The listing builds one solid part. Answer for the finished solid, in the listing's coordinates (mm). Face numbers are marked on the shaded views. A direction names the side the tool comes from. Round coordinates to 2 decimals unless told otherwise and drop trailing zeros. Loops run counter-clockwise (first coordinate to the right, second up) from the corner with the lowest first, then second, coordinate; pieces in that order, holes last. Notation, with made-up numbers: (32.25, 62) -> (44.25, 62) arc R29 ccw to (44.25, 93) -> close; hole circle Ø1 at (45.5, 44). An arc over 180 degrees is marked (long way). One line per question, with ' | ' between items.
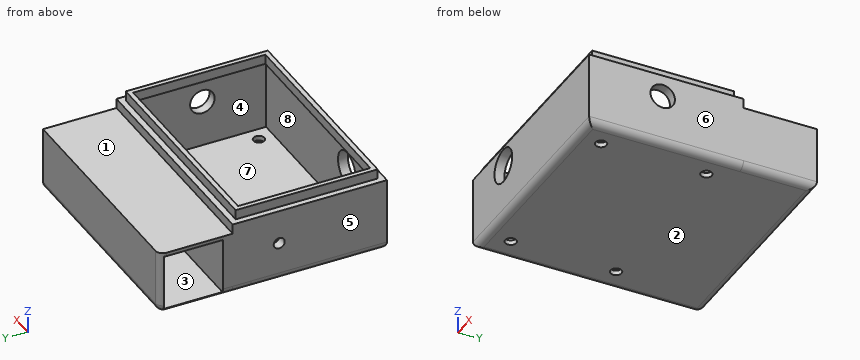
from build123d import *

# Parameters (mm, degrees)
SKETCH3_W           = 92
SKETCH3_H           = 63
SKETCH3_R           = 2.25
BOSS_EXTRUDE3_DEPTH = 30
SKETCH4_W           = 84
SKETCH4_H           = 55
CUT_EXTRUDE1_DEPTH  = 28
FILLET1_R           = 3
SKETCH5_W           = 87
SKETCH5_H           = 58
BOSS_EXTRUDE4_DEPTH = 4
SKETCH7_W           = 83
SKETCH7_H           = 54
CUT_EXTRUDE4_DEPTH  = 27
SKETCH9_R           = 7
CUT_EXTRUDE6_DEPTH  = 27
SKETCH11_R          = 5
CUT_EXTRUDE7_DEPTH  = 27
SKETCH12_R          = 2.25
CUT_EXTRUDE8_DEPTH  = 10
SKETCH13_W          = 92
SKETCH13_H          = 26
BOSS_EXTRUDE6_DEPTH = 30
SKETCH14_W          = 23
SKETCH14_H          = 24
CUT_EXTRUDE9_DEPTH  = 90
FILLET3_R           = 3
FILLET4_R           = 3


with BuildPart() as part:
    # Sketch3 → Boss-Extrude3 (new body)
    with BuildSketch(Plane.XY):
        with Locations((46, 31.5)):
            Rectangle(SKETCH3_W, SKETCH3_H)
        with Locations((82, 53)):
            Circle(SKETCH3_R, mode=Mode.SUBTRACT)
        with Locations((82, 10)):
            Circle(SKETCH3_R, mode=Mode.SUBTRACT)
        with Locations((10.5, 10)):
            Circle(SKETCH3_R, mode=Mode.SUBTRACT)
        with Locations((10.5, 53)):
            Circle(SKETCH3_R, mode=Mode.SUBTRACT)
    extrude(amount=BOSS_EXTRUDE3_DEPTH)

    # Sketch4 → Cut-Extrude1 (cut)
    with BuildSketch(Plane.XY.offset(30)):
        with Locations((46, 31.5)):
            Rectangle(SKETCH4_W, SKETCH4_H)
    extrude(amount=-CUT_EXTRUDE1_DEPTH, mode=Mode.SUBTRACT)

    # Fillet1
    fillet1_edges = [part.edges().sort_by_distance(p)[0] for p in [
        (92, 31.5, 0),
        (46, 0, 0),
        (0, 31.5, 0),
    ]]
    fillet(fillet1_edges, radius=FILLET1_R)

    # Sketch5 → Boss-Extrude4 (add)
    with BuildSketch(Plane.XY.offset(30)):
        with Locations((46, 31.5)):
            Rectangle(SKETCH5_W, SKETCH5_H)
    extrude(amount=BOSS_EXTRUDE4_DEPTH)

    # Sketch7 → Cut-Extrude4 (cut)
    with BuildSketch(Plane.XY.offset(34)):
        with Locations((46, 31.5)):
            Rectangle(SKETCH7_W, SKETCH7_H)
    extrude(amount=-CUT_EXTRUDE4_DEPTH, mode=Mode.SUBTRACT)

    # Sketch9 → Cut-Extrude6 (cut)
    with BuildSketch(Plane.XZ):
        with Locations(Location((24, 22, 0), (0, 0, 270))):
            Circle(SKETCH9_R)
    extrude(amount=-CUT_EXTRUDE6_DEPTH, mode=Mode.SUBTRACT)

    # Sketch11 → Cut-Extrude7 (cut)
    with BuildSketch(Plane(origin=(92, 0, 0), x_dir=(0, 0, -1), z_dir=(1, 0, 0))):
        with Locations((-21, 30)):
            Circle(SKETCH11_R)
    extrude(amount=-CUT_EXTRUDE7_DEPTH, mode=Mode.SUBTRACT)

    # Sketch12 → Cut-Extrude8 (cut)
    with BuildSketch(Plane.ZY):
        with Locations((16, 44)):
            Circle(SKETCH12_R)
    extrude(amount=-CUT_EXTRUDE8_DEPTH, mode=Mode.SUBTRACT)

    # Sketch13 → Boss-Extrude6 (add)
    with BuildSketch(Plane(origin=(0, 63, 0), x_dir=(1, 0, 0), z_dir=(0, 1, 0))):
        with Locations((46, -13)):
            Rectangle(SKETCH13_W, SKETCH13_H)
    extrude(amount=BOSS_EXTRUDE6_DEPTH)

    # Sketch14 → Cut-Extrude9 (cut)
    with BuildSketch(Plane.ZY):
        with Locations((13, 79)):
            Rectangle(SKETCH14_W, SKETCH14_H)
    extrude(amount=-CUT_EXTRUDE9_DEPTH, mode=Mode.SUBTRACT)

    # Fillet3
    fillet3_edges = [part.edges().sort_by_distance(p)[0] for p in [
        (46, 93, 0),
        (92, 78, 0),
    ]]
    fillet(fillet3_edges, radius=FILLET3_R)

    # Fillet4
    # the kernel refuses this fillet: 3 mm, written as the material it takes off along each edge
    with BuildSketch(Plane(origin=(0, 93, 33.5), x_dir=(0, -1, 0), z_dir=(0, 0, -1))) as fillet4_piece_1:
        with BuildLine():
            CenterArc((FILLET4_R, -FILLET4_R), FILLET4_R, 90, 90)
            Line((0, -FILLET4_R), (0, 0))
            Line((0, 0), (FILLET4_R, 0))
        make_face()
    extrude(amount=30.5, mode=Mode.SUBTRACT)
    with BuildSketch(Plane(origin=(0, 55.5, 0), x_dir=(0, 0, 1), z_dir=(0, 1, 0))) as fillet4_piece_2:
        with BuildLine():
            CenterArc((FILLET4_R, FILLET4_R), FILLET4_R, 180, 90)
            Line((0, FILLET4_R), (0, 0))
            Line((0, 0), (FILLET4_R, 0))
        make_face()
    extrude(amount=34.5, mode=Mode.SUBTRACT)
    with BuildSketch(Plane(origin=(0, 90, 3), x_dir=(0, 1, 0), z_dir=(0, 0, 1))) as fillet4_piece_3:
        with BuildLine():
            CenterArc((3 - FILLET4_R, -FILLET4_R), FILLET4_R, 0, 90)
            Line((3, -FILLET4_R), (3, 0))
            Line((3, 0), (3 - FILLET4_R, 0))
        make_face()
    revolve(axis=Axis((0, 90, 3), (-1, 0, 0)), revolution_arc=90, mode=Mode.SUBTRACT)


solid = part.part
Q1. A cutting plane is placed at D-D on z = 5. Give the vertices of the cut face in (x, y).
Numbers:
outline: (0, 0) -> (92, 0) -> (92, 93) -> (3, 93) arc R3 ccw to (0.17, 91) -> (90, 91) -> (90, 67) -> (0, 67) -> close; hole (4, 4) -> (88, 4) -> (88, 59) -> (4, 59) -> close
Q2. A cutting plane is placed at B-B on y = 10. Give the vertices of the cut face in (x, z), plus the area to 3 significant figures.
Numbers:
outline: (0, 3) arc R3 ccw to (3, 0) -> (8.25, 0) -> (8.25, 2) -> (4, 2) -> (4, 30) -> (4.5, 30) -> (4.5, 34) -> (2.5, 34) -> (2.5, 30) -> (0, 30) -> close; (12.75, 0) -> (79.75, 0) -> (79.75, 2) -> (12.75, 2) -> close; (84.25, 0) -> (89, 0) arc R3 ccw to (92, 3) -> (92, 30) -> (89.5, 30) -> (89.5, 34) -> (87.5, 34) -> (87.5, 30) -> (88, 30) -> (88, 2) -> (84.25, 2) -> close | area: 402 mm^2
Q3. A cutting plane is placed at C-C on x = 82. Give the number of separate pieces and of enclosed holes in the cut face, plus the area to 3 significant figures.
Numbers:
separate pieces: 3 | enclosed holes: 1 | area: 572 mm^2
Q4. Given pin 1 Ø1.5 at (x, z) = (91, 2) entering from -Y; pin 2 Ø4 at (x, y) = (10.5, 53) entering from -Z; pin 3 Ø4 at (x, y) = (80, 11.5) entering from +Z; pin 4 Ø3 at (y, z) = (38.5, 32.5) entering from -X, each flat-ended and moving along its own axis, determine where each tip first touches the part or whether it passes through.
Numbers:
pin 1: y = 0.01 | pin 2: through | pin 3: z = 2 | pin 4: x = 2.5
Q5. For the marked faces 1, 2, 3 and 4, determine the directions among +Z, -Z, +X, -X, +Y, -Y from which every point of the face is accessible in a straight line to the end or side of a thin tool.
Numbers:
face 1: +Z, +X, -X, +Y | face 2: -Z, +X, -X, +Y, -Y | face 3: -X | face 4: none
Q6. For a pull along X with two mould halves and no side action, classify the marked faces 5, 6, 7 and 8 as pulls with the +X half, pulls with the -X half, needs draft (parallel to the pull), parting line crosses it, or undercut.
Numbers:
face 5: pulls with the -X half | face 6: pulls with the +X half | face 7: undercut | face 8: undercut
Q7. A cutting plane is placed at A-A on x = 24. Give the vertices of the cut face in (y, z).
Numbers:
outline: (0, 3) arc R3 ccw to (3, 0) -> (90, 0) arc R3 ccw to (93, 3) -> (93, 26) -> (63, 26) -> (63, 30) -> (60.5, 30) -> (60.5, 34) -> (58.5, 34) -> (58.5, 30) -> (59, 30) -> (59, 2) -> (4, 2) -> (4, 15) -> (0, 15) -> close; (0, 29) -> (4, 29) -> (4, 30) -> (4.5, 30) -> (4.5, 34) -> (2.5, 34) -> (2.5, 30) -> (0, 30) -> close; hole (67, 1.5) -> (91, 1.5) -> (91, 24.5) -> (67, 24.5) -> close
Q8. Find the intervals of material crossed by line 1 (Y direction, x = 82.5, z = 20); line 2 (Y direction, x = 89, z = 21); line 3 (Y direction, x = 64, z = 28.5), in increasing order. Write a range as from..to.
Numbers:
line 1: 0..4, 59..67, 91..93 | line 2: 0..25, 35..67, 91..93 | line 3: 0..4, 59..63
